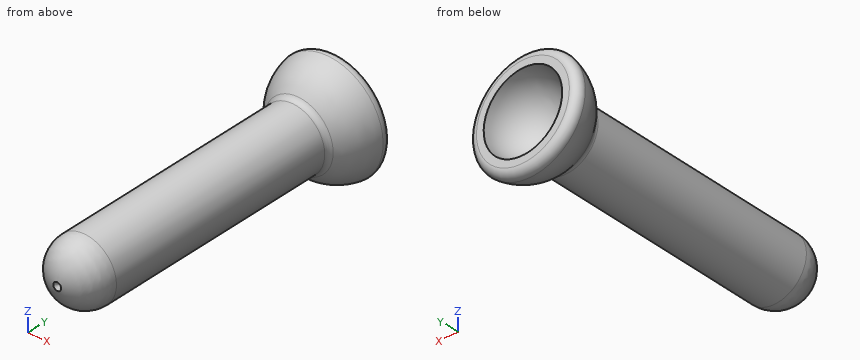
Autodesk Inventor part; units mm, degrees
ref_plane "YZ Plane" through (0, 0, 0) normal (1, 0, 0) x (0, 1, 0)
ref_plane "XZ Plane" through (0, 0, 0) normal (0, 1, 0) x (-1, 0, 0)
ref_plane "XY Plane" through (0, 0, 0) normal (0, 0, 1) x (1, 0, 0)
sketch "Sketch1" plane through (0, 0, 0) normal (1, 0, 0) x (0, 1, 0)
  line L0 (0, 0) -> (20, 0) construction
  arc A0 (20, 2.5) -> (17.5, 0) centre (20, 0) ccw
  arc A1 (19.4167, 3.451) -> (17.2678, 2.1875) centre (20, 0) ccw
  line L1 (2, 2) -> (16.8775, 2)
  line L2 (2, 2) -> (2, -2.5) construction
  arc A2 (2, 2) -> (0.0157, 0.25) centre (2, 0) ccw
  line L3 (0.25, 0) -> (0.0157, 0.25)
  line L4 (20, 0) -> (20, 2.958)
  line L5 (17.5, 0) -> (0.25, 0)
  arc A3 (20, 2.958) -> (19.4167, 3.451) centre (19.5, 2.958) ccw
  arc A4 (16.8775, 2) -> (17.2678, 2.1875) centre (16.8775, 2.5) ccw
  dimension "d0" = 20
  dimension "d1" = 5
  dimension "d2" = 7
  dimension "d3" = 2
  dimension "d4" = 2
  dimension "d5" = 0.25
  dimension "d6" = 0.25
  dimension "d7" = 1
  dimension "d8" = 1
revolve "Revolution1" add sketch "Sketch1" angle 360 about axis through (0, 0, 0) along (0, 1, 0)
properties part number "Component 4 (Pound)"
Here's how the part is built. I have some questions about the finished solid (model axes, mm). Coordinates: 2 decimals unless noted, no trailing zeros. Loops run counter-clockwise (first coordinate to the right, second up) from the corner with the lowest first, then second, coordinate; pieces in that order, holes last. Notation, with made-up numbers: (-7, 5.5) - (37, 5.5) arc R28 ccw to (37, 24.5) - close; hole circle Ø10 at (-12.5, -19). An arc over 180 degrees is marked (long way). Answer as CSV lines item,"result".
Q1. If I drill on L1, parallel to X at y = 2.75, z = 0; L2, parallel to Z at x = -1.25, y = 18.25; L3, parallel to Y at x = 0.5, z = -2, over which ranges is the centre line in solid material (lowest first)? Write a range as [from, to].
Response:
L1,"[-2, 2]"
L2,"[-2.76, -1.27], [1.27, 2.76]"
L3,"[17.12, 18.59]"
Q2. For pin 1 (3 mm diameter, centred on y = 6.5, z = -2, fed in from -X); pin 2 (2 mm diameter, centred on x = 2.5, z = -2.5, fed in from +Y); pin 3 (1.5 mm diameter, centred on y = 3.5, z = 0.5, fed in from +X); pin 4 (1 mm diameter, centred on y = 2, z = 0.5, fed in from -X), each with a flat end and sliding along its axis, tell me the tip position at first contact or that it passes through.
Response:
pin 1,"x = -1.94"
pin 2,"y = 20"
pin 3,"x = 2"
pin 4,"x = -2"
Q3. If we section it at A-A, the plane y = 8.75: Write out the boundary of the cut face in (x, z), and give its area (3 significant figures).
Response:
outline,"circle Ø4 at (0, 0)"
area,"12.6 mm2"
